from build123d import *

# Parameters (mm, degrees)
SKETCH_1_W                  = 100
SKETCH_1_H                  = 70
EXTRUDE_1_DEPTH             = 5
SKETCH_2_R                  = 3
CUT_EXTRUDE_1_DEPTH         = 10
PATTERN_LINEAR_1_COUNT      = 5
PATTERN_LINEAR_1_PITCH      = 10
PATTERN_LINEAR_1_COUNT_DIR2 = 6
PATTERN_LINEAR_1_PITCH_DIR2 = 10


with BuildPart() as part:
    # 草图1 → 凸台-拉伸1 (new, symmetric)
    with BuildSketch(Plane.XY):
        Rectangle(SKETCH_1_W, SKETCH_1_H)
    extrude(amount=EXTRUDE_1_DEPTH, both=True)

    # 草图2 → 切除-拉伸1 (cut)
    with BuildSketch(Plane.XY.offset(5)):
        with Locations((-45, 30)):
            Circle(SKETCH_2_R)
    cut_extrude_1 = extrude(amount=-CUT_EXTRUDE_1_DEPTH, mode=Mode.SUBTRACT)

    # 阵列(线性)1: Cut-Extrude 1 5 × 6
    with Locations(*[(i * PATTERN_LINEAR_1_PITCH, -j * PATTERN_LINEAR_1_PITCH_DIR2, 0) for i in range(PATTERN_LINEAR_1_COUNT) for j in range(PATTERN_LINEAR_1_COUNT_DIR2) if (i, j) != (0, 0)]):
        add(cut_extrude_1, mode=Mode.SUBTRACT)


solid = part.part
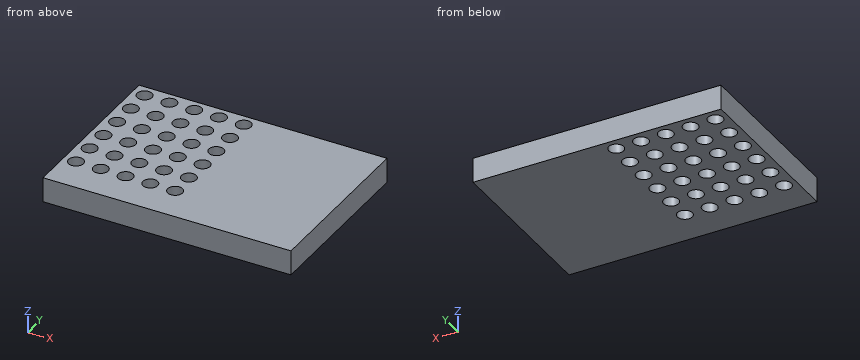
Source: CAD feature listing. Evaluate the final solid. Frame: model axes, mm. Coordinates: 2 decimals unless noted, no trailing zeros. Loops run counter-clockwise (first coordinate to the right, second up) from the corner with the lowest first, then second, coordinate; pieces in that order, holes last. Notation, with made-up numbers: (38, 19.5) - (73, 19.5) arc R16 cw to (73, 27.5) - close; hole circle Ø5 at (24.5, 40). An arc over 180 degrees is marked (long way). Return JSON: item names as keys, results as strings.
Q1. Section A-A, the plane x = -35. Return loops of the section in (y, z).
Results:
{"outline": "(-35, -5) - (-23, -5) - (-23, 5) - (-35, 5) - close; (-17, -5) - (-13, -5) - (-13, 5) - (-17, 5) - close; (-7, -5) - (-3, -5) - (-3, 5) - (-7, 5) - close; (3, -5) - (7, -5) - (7, 5) - (3, 5) - close; (13, -5) - (17, -5) - (17, 5) - (13, 5) - close; (23, -5) - (27, -5) - (27, 5) - (23, 5) - close; (33, -5) - (35, -5) - (35, 5) - (33, 5) - close"}
Q2. Material intervals for line 1 along X through (y, z) = (29.5, -4); line 2 along X through (y, z) = (-12, 1.75), sorted ascending.
Results:
{"line 1": "-50 to -47.96, -42.04 to -37.96, -32.04 to -27.96, -22.04 to -17.96, -12.04 to -7.96, -2.04 to 50", "line 2": "-50 to -47.24, -42.76 to -37.24, -32.76 to -27.24, -22.76 to -17.24, -12.76 to -7.24, -2.76 to 50"}
Q3. Section C-C, the plane y = -10. Return loops of the section in (x, z).
Results:
{"outline": "(-50, -5) - (-48, -5) - (-48, 5) - (-50, 5) - close; (-42, -5) - (-38, -5) - (-38, 5) - (-42, 5) - close; (-32, -5) - (-28, -5) - (-28, 5) - (-32, 5) - close; (-22, -5) - (-18, -5) - (-18, 5) - (-22, 5) - close; (-12, -5) - (-8, -5) - (-8, 5) - (-12, 5) - close; (-2, -5) - (50, -5) - (50, 5) - (-2, 5) - close"}
Q4. Section B-B, the plane z = -0.5. Give the number of separate pieces and of enclosed holes in the cut face, plus the area to 3 significant figures.
Results:
{"separate pieces": "1", "enclosed holes": "30", "area": "6,150 mm2"}
